Read the model definition and answer for the solid it produces. Units are mm, in the model's axes. A direction names the side the tool comes from. Coordinates: 2 decimals unless noted, no trailing zeros. Loops run counter-clockwise (first coordinate to the right, second up) from the corner with the lowest first, then second, coordinate; pieces in that order, holes last. Notation, with made-up numbers: (9.5, -35.75) -> (55.5, -35.75) arc R21 cw to (55.5, -6.75) -> close; hole circle Ø8 at (61.5, -21). An arc over 180 degrees is marked (long way). Answer as a JSON object with one key per item and string values. Group by question number.
1) Consider probe 1 along Z at (x, y) = (224, 1.5); probe 2 along Z at (x, y) = (56.5, 1.25); probe 3 along X at (y, z) = (2.8, -85). Determine where each line is inside the solid, lowest interval first. Write a range as [from, to].
2) Flat-ended cylindrical pins translate along their axes: P1, Ø2, axis at y = 0.5, z = -108, coming from the +X side; P2, Ø1.5, axis at y = 2, z = -163, coming from the -X side; P3, Ø15.5, axis at x = 314, z = -137, coming from the +Y side; P4, Ø2.5, axis at x = 182, z = -32, coming from the -Y side. Find the tip coordinate at first contact, or state that the pin passes through.
3) Determine the mould class of faces 1 (the face through (308, 3.5, -136)), 2 (the face through (0, 2, -86)), 3 (the face through (85, 1, -155)) for opening direction Z: released by +Z, released by -Z, zero draft, split by the parting line, or undercut.
4) Which of the six approach directions +Z, -Z, +X, -X, +Y, -Y give full straight-line access (tool end or side, diameter ignored) to faces 4 (the face through (191.62, 1.96, -25.54)), 5 (the face through (70, 2, -99)), 6 (the face through (308, 3.5, -85))?
5) Section A-A, the plane y = 1.5 is taken. Count the separate pieces of the cut face and the enclosed holes in it, plus the area to 3 significant figures.
6) Section B-B, the plane x = 277.5 is taken. Give the vertices of the cut face in (y, z).
from build123d import *

# Parameters (mm, degrees)
BOSS_EXTRUDE1_DEPTH      = 5
BOSS_EXTRUDE1_DEPTH_BACK = 1
SKETCH1_R                = 2
SKETCH3_R                = 1.5
SKETCH3_W                = 8
SKETCH3_H                = 14
SKETCH3_W_2              = 60
SKETCH3_H_2              = 6
SKETCH3_W_3              = 30
CUT_EXTRUDE2_DEPTH       = 382.529815349
FILLET1_R                = 5
FILLET2_R                = 10
FILLET3_R                = 5
FILLET4_R                = 10
FILLET5_R                = 5
FILLET6_R                = 5
FILLET7_R                = 5
FILLET8_R                = 5
FILLET9_R                = 5
FILLET10_R               = 5
FILLET11_R               = 5
FILLET12_R               = 5
CUT_EXTRUDE3_DEPTH       = 2
SKETCH5_W                = 23
SKETCH5_H                = 14
CUT_EXTRUDE4_DEPTH       = 1.5


with BuildPart() as part:
    # Sketch1 → Boss-Extrude1 (new, two sides: drawn at the far end of the back side and taken through both)
    with BuildSketch(Plane(origin=(0, 0, 0), x_dir=(1, 0, 0), z_dir=(0, 1, 0)).offset(-BOSS_EXTRUDE1_DEPTH_BACK)):
        with BuildLine():
            ThreePointArc((0, 20), (5.857864376, 5.857864376), (20, 0))
            Line((20, 0), (50, 0))
            Line((50, 0), (50, 15))
            Line((50, 15), (120, 15))
            Line((120, 15), (120, 0))
            Line((120, 0), (174.516287626, 0))
            ThreePointArc((174.516287626, 0), (184.152968357, 3.50502786), (189.286071162, 12.382082068))
            Line((189.286071162, 12.382082068), (194.016707233, 39.071410209))
            ThreePointArc((194.016707233, 39.071410209), (197.438775769, 44.989446348), (203.86322959, 47.326131588))
            Line((203.86322959, 47.326131588), (275.479841954, 47.326131588))
            Line((275.479841954, 47.326131588), (281.957258661, 47.326131588))
            ThreePointArc((281.957258661, 47.326131588), (289.464356355, 43.932453122), (291.876118892, 36.05482843))
            ThreePointArc((291.876118892, 36.05482843), (289.726144633, 21.493661084), (287.021151563, 7.025316456))
            ThreePointArc((287.021151563, 7.025316456), (286.072411794, 2.570993654), (285.071048277, -1.871794872))
            Line((285.071048277, -1.871794872), (328.414372402, -3))
            ThreePointArc((328.414372402, -3), (329.306211212, 0.398467763), (330.162883312, 3.805970149))
            ThreePointArc((330.162883312, 3.805970149), (340, 85), (330.162883312, 166.194029851))
            ThreePointArc((330.162883312, 166.194029851), (329.306211212, 169.601532237), (328.414372402, 173))
            Line((328.414372402, 173), (285.071048277, 171.871794872))
            ThreePointArc((285.071048277, 171.871794872), (286.072411794, 167.429006346), (287.021151563, 162.974683544))
            ThreePointArc((287.021151563, 162.974683544), (289.726144633, 148.506338916), (291.876118892, 133.94517157))
            ThreePointArc((291.876118892, 133.94517157), (289.464356355, 126.067546878), (281.957258661, 122.673868412))
            Line((281.957258661, 122.673868412), (275.479841954, 122.673868412))
            Line((275.479841954, 122.673868412), (203.86322959, 122.673868412))
            ThreePointArc((203.86322959, 122.673868412), (197.438775769, 125.010553652), (194.016707233, 130.928589791))
            Line((194.016707233, 130.928589791), (189.286071162, 157.617917932))
            ThreePointArc((189.286071162, 157.617917932), (184.152968357, 166.49497214), (174.516287626, 170))
            Line((174.516287626, 170), (120, 170))
            Line((120, 170), (120, 155))
            Line((120, 155), (50, 155))
            Line((50, 155), (50, 170))
            Line((50, 170), (20, 170))
            ThreePointArc((20, 170), (5.857864376, 164.142135624), (0, 150))
            Line((0, 150), (0, 85))
            Line((0, 85), (0, 20))
        make_face()
        with Locations(Location((77, 23, 0), (0, 0, 270))):
            Circle(SKETCH1_R, mode=Mode.SUBTRACT)
        with Locations(Location((77, 37, 0), (0, 0, 270))):
            Circle(SKETCH1_R, mode=Mode.SUBTRACT)
        with Locations(Location((93, 23, 0), (0, 0, 270))):
            Circle(SKETCH1_R, mode=Mode.SUBTRACT)
        with Locations(Location((93, 37, 0), (0, 0, 270))):
            Circle(SKETCH1_R, mode=Mode.SUBTRACT)
        with Locations(Location((77, 133, 0), (0, 0, 270))):
            Circle(SKETCH1_R, mode=Mode.SUBTRACT)
        with Locations(Location((77, 147, 0), (0, 0, 270))):
            Circle(SKETCH1_R, mode=Mode.SUBTRACT)
        with Locations(Location((93, 133, 0), (0, 0, 270))):
            Circle(SKETCH1_R, mode=Mode.SUBTRACT)
        with Locations(Location((93, 147, 0), (0, 0, 270))):
            Circle(SKETCH1_R, mode=Mode.SUBTRACT)
    extrude(amount=BOSS_EXTRUDE1_DEPTH + BOSS_EXTRUDE1_DEPTH_BACK)

    # Sketch3 → Cut-Extrude2 (cut, through all)
    with BuildSketch(Plane(origin=(0, 5, 0), x_dir=(1, 0, 0), z_dir=(0, 1, 0))):
        with Locations(Location((304, 34, 0), (0, 0, 270))):
            Circle(SKETCH3_R)
        with Locations(Location((304, 51, 0), (0, 0, 270))):
            Circle(SKETCH3_R)
        with Locations((324, 51)):
            Rectangle(SKETCH3_W, SKETCH3_H)
        with Locations((324, 34)):
            Rectangle(SKETCH3_W, SKETCH3_H)
        with Locations(Location((304, 68, 0), (0, 0, 270))):
            Circle(SKETCH3_R)
        with Locations(Location((304, 85, 0), (0, 0, 270))):
            Circle(SKETCH3_R)
        with Locations(Location((304, 102, 0), (0, 0, 270))):
            Circle(SKETCH3_R)
        with Locations((324, 102)):
            Rectangle(SKETCH3_W, SKETCH3_H)
        with Locations((324, 119)):
            Rectangle(SKETCH3_W, SKETCH3_H)
        with Locations((324, 85)):
            Rectangle(SKETCH3_W, SKETCH3_H)
        with Locations((324, 68)):
            Rectangle(SKETCH3_W, SKETCH3_H)
        with Locations((324, 136)):
            Rectangle(SKETCH3_W, SKETCH3_H)
        with Locations(Location((304, 136, 0), (0, 0, 270))):
            Circle(SKETCH3_R)
        with Locations(Location((304, 119, 0), (0, 0, 270))):
            Circle(SKETCH3_R)
        with Locations(Location((247, 85, 0), (0, 0, 270))):
            Circle(SKETCH3_R)
        with Locations(Location((287, 85, 0), (0, 0, 270))):
            Circle(SKETCH3_R)
        with Locations((70, 68)):
            Rectangle(SKETCH3_W_2, SKETCH3_H_2)
        with Locations((70, 102)):
            Rectangle(SKETCH3_W_2, SKETCH3_H_2)
        with Locations((215, 103)):
            Rectangle(SKETCH3_W_3, SKETCH3_H_2)
        with Locations((215, 67)):
            Rectangle(SKETCH3_W_3, SKETCH3_H_2)
        with Locations(Location((10, 138, 0), (0, 0, 270))):
            Circle(SKETCH3_R)
        with Locations(Location((10, 32, 0), (0, 0, 270))):
            Circle(SKETCH3_R)
        with Locations(Location((182, 138, 0), (0, 0, 270))):
            Circle(SKETCH3_R)
        with Locations(Location((182, 32, 0), (0, 0, 270))):
            Circle(SKETCH3_R)
    extrude(amount=-CUT_EXTRUDE2_DEPTH, mode=Mode.SUBTRACT)

    # Fillet1
    fillet1_edges = [part.edges().sort_by_distance(p)[0] for p in [
        (285.071048277, 2, -171.871794872),
    ]]
    fillet(fillet1_edges, radius=FILLET1_R)

    # Fillet2
    fillet2_edges = [part.edges().sort_by_distance(p)[0] for p in [
        (328.414372402, 2.5, -173),
    ]]
    fillet(fillet2_edges, radius=FILLET2_R)

    # Fillet3
    fillet3_edges = [part.edges().sort_by_distance(p)[0] for p in [
        (285.071048277, 2, 1.871794872),
    ]]
    fillet(fillet3_edges, radius=FILLET3_R)

    # Fillet4
    fillet4_edges = [part.edges().sort_by_distance(p)[0] for p in [
        (328.414372402, 2.5, 3),
    ]]
    fillet(fillet4_edges, radius=FILLET4_R)

    # Fillet5
    fillet5_edges = [part.edges().sort_by_distance(p)[0] for p in [
        (50, 2, -15),
    ]]
    fillet(fillet5_edges, radius=FILLET5_R)

    # Fillet6
    fillet6_edges = [part.edges().sort_by_distance(p)[0] for p in [
        (120, 2, -15),
    ]]
    fillet(fillet6_edges, radius=FILLET6_R)

    # Fillet7
    fillet7_edges = [part.edges().sort_by_distance(p)[0] for p in [
        (120, 2, -155),
    ]]
    fillet(fillet7_edges, radius=FILLET7_R)

    # Fillet8
    fillet8_edges = [part.edges().sort_by_distance(p)[0] for p in [
        (50, 2, -155),
    ]]
    fillet(fillet8_edges, radius=FILLET8_R)

    # Fillet9
    fillet9_edges = [part.edges().sort_by_distance(p)[0] for p in [
        (50, 2, -170),
    ]]
    fillet(fillet9_edges, radius=FILLET9_R)

    # Fillet10
    fillet10_edges = [part.edges().sort_by_distance(p)[0] for p in [
        (120, 2, -170),
    ]]
    fillet(fillet10_edges, radius=FILLET10_R)

    # Fillet11
    fillet11_edges = [part.edges().sort_by_distance(p)[0] for p in [
        (50, 2, 0),
    ]]
    fillet(fillet11_edges, radius=FILLET11_R)

    # Fillet12
    fillet12_edges = [part.edges().sort_by_distance(p)[0] for p in [
        (120, 2, 0),
    ]]
    fillet(fillet12_edges, radius=FILLET12_R)

    # Sketch4 → Cut-Extrude3 (cut)
    with BuildSketch(Plane(origin=(0, 5, 0), x_dir=(1, 0, 0), z_dir=(0, 1, 0))):
        with BuildLine():
            Line((74, 46.5), (96, 46.5))
            ThreePointArc((96, 46.5), (97.414213562, 45.914213562), (98, 44.5))
            Line((98, 44.5), (98, 15))
            Line((98, 15), (72, 15))
            Line((72, 15), (72, 44.5))
            ThreePointArc((72, 44.5), (72.585786438, 45.914213562), (74, 46.5))
        make_face()
        with BuildLine():
            Line((72, 155), (98, 155))
            Line((98, 155), (98, 125.5))
            ThreePointArc((98, 125.5), (97.414213562, 124.085786438), (96, 123.5))
            Line((96, 123.5), (74, 123.5))
            ThreePointArc((74, 123.5), (72.585786438, 124.085786438), (72, 125.5))
            Line((72, 125.5), (72, 155))
        make_face()
    extrude(amount=-CUT_EXTRUDE3_DEPTH, mode=Mode.SUBTRACT)

    # Sketch5 → Cut-Extrude4 (cut)
    with BuildSketch(Plane(origin=(0, 5, 0), x_dir=(1, 0, 0), z_dir=(0, 1, 0))):
        with Locations((308.5, 51)):
            Rectangle(SKETCH5_W, SKETCH5_H)
        with Locations((308.5, 34)):
            Rectangle(SKETCH5_W, SKETCH5_H)
        with Locations((308.5, 68)):
            Rectangle(SKETCH5_W, SKETCH5_H)
        with Locations((308.5, 85)):
            Rectangle(SKETCH5_W, SKETCH5_H)
        with Locations((308.5, 102)):
            Rectangle(SKETCH5_W, SKETCH5_H)
        with Locations((308.5, 119)):
            Rectangle(SKETCH5_W, SKETCH5_H)
        with Locations((308.5, 136)):
            Rectangle(SKETCH5_W, SKETCH5_H)
    extrude(amount=-CUT_EXTRUDE4_DEPTH, mode=Mode.SUBTRACT)


solid = part.part
Determined:
{
 "1": {"probe 1": "[-122.67, -106], [-100, -70], [-64, -47.33]", "probe 2": "[-155, -105], [-99, -71], [-65, -15]", "probe 3": "[0, 245.5], [248.5, 285.5], [288.5, 302.5], [305.5, 320], [328, 340]"},
 "2": {"P1": "x = 339.29", "P2": "x = 4.19", "P3": "y = 5", "P4": "through"},
 "3": {"face 1": "undercut", "face 2": "zero draft", "face 3": "released by -Z"},
 "4": {"face 4": "+Z, +Y, -Y", "face 5": "+Y, -Y", "face 6": "+Y"},
 "5": {"separate pieces": "1", "enclosed holes": "32", "area": "43,700 mm²"},
 "6": {"outline": "(-1, -122.67) -> (5, -122.67) -> (5, -47.33) -> (-1, -47.33) -> close"}
}
